Geometry: see drawing. Coordinates: mm, zero at the bounding-box minimum. A direction names the side the tool comes from. Give positions to 0.01 mm unless a question says otherwise; leave off trailing zeros. Order: outer loops, then holes, each group sorted by start corner. A loop starts at its lowest first (then second) coordinate and runs counter-clockwise, first axis right, second up. Notation, with made-up numbers: (-11, 23.5) - (3, 23.5) arc R27 cw to (3, 61.5) - close; hole circle Ø5 at (-5.5, 63). An arc over 180 degrees is marked (long way). One line per question, with ' | ' between items. Start each with the question number.
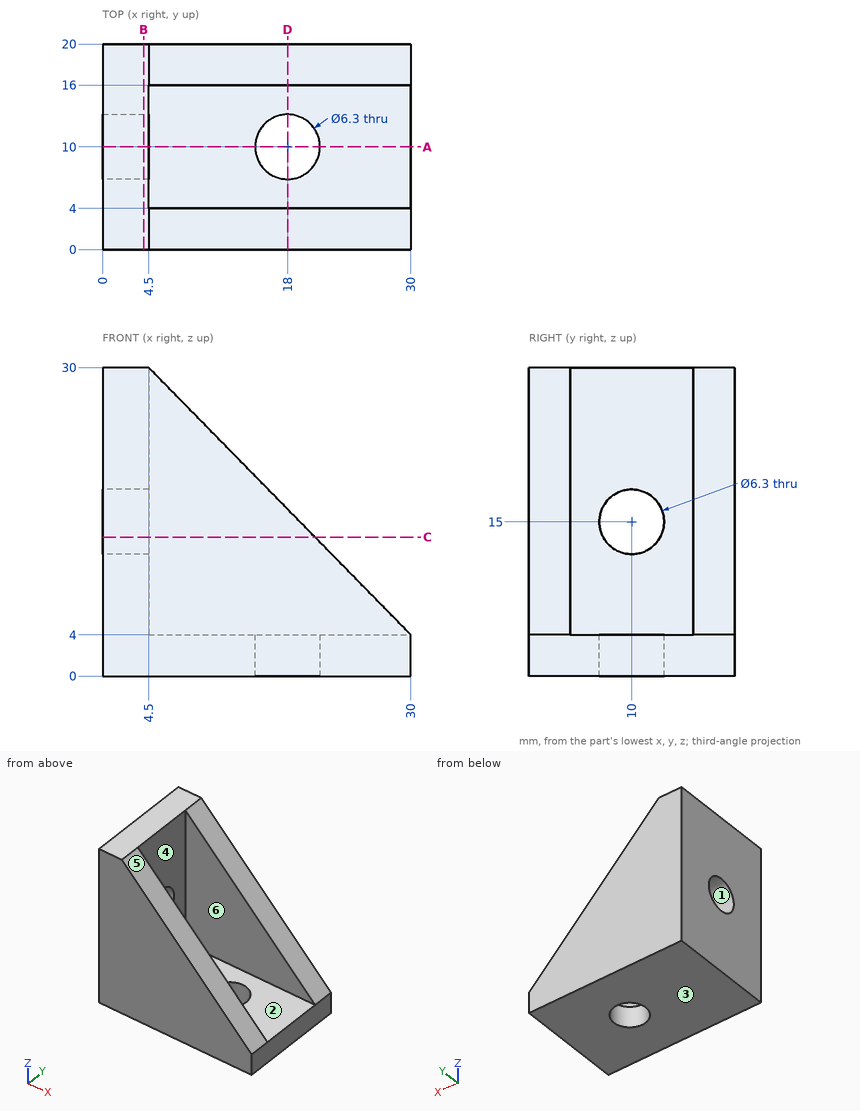
(1) Cut plane D-D, the plane x = 18. Return the cut outline in (y, z), plus the area to 3 significant figures.
(2) Access query for the marked faces 5 and 6. Directions: +Z, -Z, +X, -X, +Y, -Y. A direction counts if a zero-diameter tool reaches every point of the face in a straight line with its end or side. Return the directions, or none.
(3) Contact query for flat-ended pins moving along their axis: P1, Ø9.5, axis at y = 7, z = 18, coming from the +X side; P2, Ø3, axis at x = 13.5, y = 12, coming from the +Z side; P3, Ø5.5, axis at x = 18, y = 10, coming from the +Z side. Output: stop coordinate, or through.
(4) Material intervals for line 1 along Y through (x, z) = (2.9, 15); line 2 along Z through (x, y) = (2.9, 10); line 3 along Y through (x, z) = (16.25, 16.5), sorted ascending. Write a range as from..to.
(5) Cut plane C-C, the plane z = 13.5. Return the cut outline in (x, y).
(6) Cut plane B-B, the plane x = 4. Return the cut outline in (y, z), plus the area to 3 significant figures.
(7) Cut plane A-A, the plane y = 10. Return the cut outline in (x, z), plus the area to 3 significant figures.
(8) Pull-direction query (Z, two-part tool) for the marked faces 1, 2, 3 and 4; classes: +Z half, -Z half, draft (parallel to the pull), parting line (faces both ways), or undercut.
Results are:
1) outline: (0, 0) - (6.85, 0) - (6.85, 4) - (4, 4) - (4, 16.24) - (0, 16.24) - close; (13.15, 0) - (20, 0) - (20, 16.24) - (16, 16.24) - (16, 4) - (13.15, 4) - close | area: 153 mm2
2) face 5: +Z, +X, +Y, -Y | face 6: +Z, +X
3) P1: x = 19.88 | P2: z = 4 | P3: through
4) line 1: 0..6.85, 13.15..20 | line 2: 0..11.85, 18.15..30 | line 3: 0..4, 16..20
5) outline: (0, 0) - (20.68, 0) - (20.68, 4) - (4.5, 4) - (4.5, 7.23) - (0, 7.23) - close; (0, 12.77) - (4.5, 12.77) - (4.5, 16) - (20.68, 16) - (20.68, 20) - (0, 20) - close
6) outline: (0, 0) - (20, 0) - (20, 30) - (0, 30) - close; hole circle Ø6.3 at (10, 15) | area: 569 mm2
7) outline: (0, 0) - (14.85, 0) - (14.85, 4) - (4.5, 4) - (4.5, 11.85) - (0, 11.85) - close; (0, 18.15) - (4.5, 18.15) - (4.5, 30) - (0, 30) - close; (21.15, 0) - (30, 0) - (30, 4) - (21.15, 4) - close | area: 183 mm2
8) face 1: undercut | face 2: +Z half | face 3: -Z half | face 4: draft
